Geometry: final body of the model. Coordinates: model frame, mm. A direction names the side the tool comes from. Round coordinates to 2 decimals unless told otherwise and drop trailing zeros. Loops run counter-clockwise (first coordinate to the right, second up) from the corner with the lowest first, then second, coordinate; pieces in that order, holes last. Notation, with made-up numbers: M -17,-29 L 18,-29 A34 cw 18,6 Z; hole C 55.5,33 d1. An arc over 180 degrees is marked long. Answer as a JSON object with one key per item and string values.
```python
from build123d import *

# Parameters (mm, degrees)
F1_DEPTH     = 3.81
F2_R         = 4.2924717139
F3_R         = 2.032
F4_T4_DEPTH  = 27.583079529
F5_R         = 2.032
F6_T1_DEPTH  = 18.831700203
F6_T6_DEPTH  = 29.7046687957
F6_T11_DEPTH = 27.9890917976


# Not quite as in the source:
# - a fillet or chamfer that OpenCascade refuses, or shapes differently, is made with other operations: its cross-section is extruded or revolved along the edge and cut away or added


with BuildPart() as f1:
    # F0 (on Right) → F1 (new body)
    with BuildSketch(Plane.YZ):
        Polygon((-48.4873987734, 60.7866533101), (-48.4873987734, 33.8229238987), (-48.4873987734, 28.1463507563), (-48.4873987734, -63.624933362), (-48.9604510367, -70.247605443), (27.200255543, -70.247605443), (27.200255543, -63.624933362), (9.6974885091, -63.624933362), (19.158443436, -14.901005663), (29.0924459696, 0), (29.0924459696, 8.7513877079), (10.1705361158, 13.954914175), (0, 54.6370334923), (22.4697776139, 64.5710304379), (17.9654553963, 74.7593885665), align=None)
    extrude(amount=F1_DEPTH)

    # F2
    f2_edges = [f1.edges().sort_by_distance(p)[0] for p in [
        (1.905, 22.469778, 64.57103),
    ]]
    fillet(f2_edges, radius=F2_R)

    # F3
    f3_edges = [f1.edges().sort_by_distance(p)[0] for p in [
        (3.81, 18.448872, -63.624933),
    ]]
    fillet(f3_edges, radius=F3_R)

    # F4: fillet of radius 2.032 on 1 edges, made by hand


with BuildPart() as f4_tool2:
    # F4_s3 → F4_t4 (new body)
    with BuildSketch(Plane.XZ.offset(-32.2404117906)):
        with BuildLine():
            ThreePointArc((1.778, -63.624933362), (0.508, -64.296954195), (0, -65.640995861))
            Line((0, -65.640995861), (0, -63.624933362))
            Line((0, -63.624933362), (1.778, -63.624933362))
        make_face()
    extrude(amount=F4_T4_DEPTH)

    split(bisect_by=Plane(origin=(0, 21.2506127093, -4.1263317328), x_dir=(1, 0, 0), z_dir=(0, 0.981664966, -0.1906145181)), keep=Keep.TOP)


with BuildPart() as f1_1:
    add(f1.part)

    # F4_t1: cut F4_tool2
    add(f4_tool2.part, mode=Mode.SUBTRACT)

    # F5
    f5_edges = [f1_1.edges().sort_by_distance(p)[0] for p in [
        (0, 24.125445, -7.450503),
        (0, 29.092446, 4.375694),
        (0, 19.631491, 11.353151),
    ]]
    fillet(f5_edges, radius=F5_R)

    # F6: fillet of radius 2.032 on 3 edges, made by hand

    # F6_s2 → F6_t1 (cut)
    with BuildSketch(Plane.XY.offset(-5.0401562476)):
        with BuildLine():
            ThreePointArc((3.81, 27.0763834706), (3.302, 28.4204251366), (2.032, 29.0924459696))
            Line((2.032, 29.0924459696), (2.03708, 29.1327672196))
            ThreePointArc((2.03708, 29.1327672196), (2.921, 29.1330859696), (3.81, 29.1330859696))
            Line((3.81, 29.1330859696), (3.85064, 29.0924459696))
            Line((3.85064, 29.0924459696), (3.85064, 27.0763834706))
            Line((3.85064, 27.0763834706), (3.81, 27.0763834706))
        make_face()
    extrude(amount=F6_T1_DEPTH, mode=Mode.SUBTRACT)


with BuildPart() as f6_tool4:
    # F6_s5 → F6_t6 (new body)
    with BuildSketch(Plane(origin=(0, 29.6693335374, -8.1590686942), x_dir=(1, 0, 0), z_dir=(0, -0.9642053764, 0.2651565426))):
        with BuildLine():
            ThreePointArc((3.81, 14.1361249687), (3.302, 15.4801666347), (2.032, 16.1521874677))
            Line((2.032, 16.1521874677), (2.03708, 16.1925087177))
            ThreePointArc((2.03708, 16.1925087177), (2.921, 16.1928274677), (3.81, 16.1928274677))
            Line((3.81, 16.1928274677), (3.85064, 16.1521874677))
            Line((3.85064, 16.1521874677), (3.85064, 14.1361249687))
            Line((3.85064, 14.1361249687), (3.81, 14.1361249687))
        make_face()
    extrude(amount=F6_T6_DEPTH)

    split(bisect_by=Plane(origin=(0, 12.8557795978, 3.213946886), x_dir=(1, 0, 0), z_dir=(0, 0.9701424649, 0.2425357661)), keep=Keep.TOP)


with BuildPart() as f1_2:
    add(f1_1.part)

    # F6_t3: cut F6_tool4
    add(f6_tool4.part, mode=Mode.SUBTRACT)


with BuildPart() as f6_tool9:
    # F6_s10 → F6_t11 (new body)
    with BuildSketch(Plane(origin=(0, -3.7782576637, -5.6673872039), x_dir=(1, 0, 0), z_dir=(0, 0.5547001482, 0.8320503263))):
        with BuildLine():
            ThreePointArc((2.032, 24.206379163), (3.302, 23.53435833), (3.81, 22.190316664))
            Line((3.81, 22.190316664), (3.85064, 22.190316664))
            Line((3.85064, 22.190316664), (3.85064, 24.206379163))
            Line((3.85064, 24.206379163), (3.81, 24.247019163))
            ThreePointArc((3.81, 24.247019163), (2.921, 24.247019163), (2.03708, 24.246700413))
            Line((2.03708, 24.246700413), (2.032, 24.206379163))
        make_face()
    extrude(amount=F6_T11_DEPTH)

    split(bisect_by=Plane(origin=(0, 21.2506127093, -4.1263317328), x_dir=(1, 0, 0), z_dir=(0, 0.981664966, -0.1906145181)), keep=Keep.TOP)


with BuildPart() as f1_3:
    add(f1_2.part)

    # F6_t8: cut F6_tool9
    add(f6_tool9.part, mode=Mode.SUBTRACT)


solid = f1_3.part
```
1) First-contact query: pin 1 (2 mm diameter, centred on x = 2.5, z = 39, fed in from +Y); pin 2 (1.1 mm diameter, centred on x = 1.5, z = 3, fed in from -Y); pin 3 (1 mm diameter, centred on y = -8.5, z = 58, fed in from -X); pin 4 (1.9 mm diameter, centred on x = 3, z = -66, fed in from +Y). Flat tips, straight axial feed; report the tip coordinate or a pass-through.
Geometry results:
{"pin 1": "y = 4.16", "pin 2": "y = -48.49", "pin 3": "x = 0", "pin 4": "y = 27.2"}
2) Cut plane A-A on y = 2. Return the cut outline in (x, z), and give its area (3 significant figures).
Geometry results:
{"outline": "M 0,-70.25 L 3.81,-70.25 L 3.81,46.64 L 0,46.64 Z; M 0,55.52 L 3.81,55.52 L 3.81,71.4 L 0,71.4 Z", "area": "506 mm2"}
3) Pull-direction query (Z, two-part tool) for faces 1 (the face through (1.88, -48.72, -66.89)), 2 (the face through (1.932, 20.794, 65.169)), 3 (the face through (3.81, -20, 3)); classes: +Z half, -Z half, draft (parallel to the pull), parting line (faces both ways), or undercut.
Geometry results:
{"face 1": "+Z half", "face 2": "undercut", "face 3": "draft"}
4) Set-up query: faces 4 (the face through (2, -48.487, -1)), 5 (the face through (1.88, 9.14, 58.68)), 6 (the face through (0.61, 19.35, 10.83)). Return all of +Z, -Z, +X, -X, +Y, -Y with unobstructed straight access to the full face (end or side cutting, diameter ignored); none if empty.
Geometry results:
{"face 4": "+Z, +X, -X, -Y", "face 5": "+X, -X, +Y", "face 6": "-X, +Y"}
5) Cut plane D-D on z = 36. Return the cut outline in (x, y).
Geometry results:
{"outline": "M 0,-48.49 L 3.81,-48.49 L 3.81,4.66 L 0,4.66 Z"}
6) Cut plane B-B on x = 0.6. Return the cut outline in (y, z).
Geometry results:
{"outline": "M -48.96,-70.25 L 27.2,-70.25 L 27.2,-64.2 L 9.59,-64.2 L 19.45,-13.4 L 28.5,0.18 L 28.5,8.3 L 10.33,13.3 L 0,54.64 L 18.54,62.84 A4.29 ccw 20.73,68.5 L 17.97,74.76 L -48.49,60.79 L -48.49,-63.62 Z"}
7) Cut plane C-C on y = 15. Count the separate pieces of the cut face and the enclosed holes in it, and give its area (3 significant figures).
Geometry results:
{"separate pieces": "3", "enclosed holes": "0", "area": "257 mm2"}
8) Line query: probe 1 along Y at (x, z) = (2.2, 4); probe 2 along Z at (x, y) = (3.15, -39.5); probe 3 along Z at (x, y) = (0.75, -31). Output: solid intervals per line, ascending.
Geometry results:
{"probe 1": "-48.49 to 29.06", "probe 2": "-70.25 to 62.68", "probe 3": "-70.25 to 64.46"}
